from build123d import *

# Parameters (mm, degrees)
SKETCH1_W           = 65
SKETCH1_H           = 51.65
BOSS_EXTRUDE1_DEPTH = 1
CHAMFER1_SIZE       = 5
CUT_EXTRUDE2_REACH  = 43.523
SKETCH2_R           = 1.75
SKETCH3_W           = 25.5
SKETCH3_H           = 1
BOSS_EXTRUDE3_DEPTH = 1
CUT_EXTRUDE3_REACH  = 44.152
SKETCH4_R           = 0.5
LPATTERN1_COUNT     = 6
LPATTERN1_PITCH     = 2.54
LPATTERN1_COL_COUNT = 5
LPATTERN1_COL_PITCH = 2.54
SKETCH5_W           = 9
SKETCH5_H           = 3.35
BOSS_EXTRUDE4_DEPTH = 1
CUT_EXTRUDE4_DEPTH  = 0.2


with BuildPart() as part:
    # Sketch1 → Boss-Extrude1 (new body)
    with BuildSketch(Plane(origin=(0, 0, 0), x_dir=(1, 0, 0), z_dir=(0, 1, 0))):
        Rectangle(SKETCH1_W, SKETCH1_H)
    extrude(amount=BOSS_EXTRUDE1_DEPTH)

    # Chamfer1
    chamfer1_edges = [part.edges().sort_by_distance(p)[0] for p in [
        (-32.5, 0.5, -25.825),
        (32.5, 0.5, -25.825),
        (32.5, 0.5, 25.825),
        (-32.5, 0.5, 25.825),
    ]]
    chamfer(chamfer1_edges, length=CHAMFER1_SIZE)

    # Sketch2 → Cut-Extrude2 (cut, up to next)
    with BuildSketch(Plane(origin=(0, 0, 0), x_dir=(1, 0, 0), z_dir=(0, 1, 0)), mode=Mode.PRIVATE) as cut_extrude2_sk1:
        with Locations(Location((-25.3, 18.625, 0), (0, 0, 270))):
            Circle(SKETCH2_R)
    cut_extrude2_tool1 = extrude(cut_extrude2_sk1.sketch, amount=CUT_EXTRUDE2_REACH, mode=Mode.PRIVATE) & part.part
    # Sketch2 → Cut-Extrude2 (cut, up to next)
    with BuildSketch(Plane(origin=(0, 0, 0), x_dir=(1, 0, 0), z_dir=(0, 1, 0)), mode=Mode.PRIVATE) as cut_extrude2_sk2:
        with Locations(Location((25.3, 18.625, 0), (0, 0, 270))):
            Circle(SKETCH2_R)
    cut_extrude2_tool2 = extrude(cut_extrude2_sk2.sketch, amount=CUT_EXTRUDE2_REACH, mode=Mode.PRIVATE) & part.part
    add(cut_extrude2_tool1.solids().sort_by_distance((-25.3, 0, -18.625))[0], mode=Mode.SUBTRACT)
    add(cut_extrude2_tool2.solids().sort_by_distance((25.3, 0, -18.625))[0], mode=Mode.SUBTRACT)

    # Sketch3 → Boss-Extrude3 (add)
    with BuildSketch(Plane(origin=(0, 1, 0), x_dir=(1, 0, 0), z_dir=(0, 1, 0))):
        with Locations((0, 26.325)):
            Rectangle(SKETCH3_W, SKETCH3_H)
    extrude(amount=-BOSS_EXTRUDE3_DEPTH)

    # Sketch4 → Cut-Extrude3 (cut, up to next)
    with BuildSketch(Plane(origin=(0, 1, 0), x_dir=(1, 0, 0), z_dir=(0, 1, 0)), mode=Mode.PRIVATE) as cut_extrude3_sk1:
        with Locations(Location((-1.27, 25.825, 0), (0, 0, 270))):
            Circle(SKETCH4_R)
    cut_extrude3_tool1 = extrude(cut_extrude3_sk1.sketch, amount=-CUT_EXTRUDE3_REACH, mode=Mode.PRIVATE) & part.part
    cut_extrude3 = cut_extrude3_tool1.solids().sort_by_distance((-1.27, 1, -25.825))[0]
    add(cut_extrude3, mode=Mode.SUBTRACT)

    # LPattern1: Cut-Extrude3 ×6
    with Locations(*[(i * LPATTERN1_PITCH, 0, 0) for i in range(1, LPATTERN1_COUNT)]):
        add(cut_extrude3, mode=Mode.SUBTRACT)

    # LPattern1 col: Cut-Extrude3 ×5
    with Locations(*[(-i * LPATTERN1_COL_PITCH, 0, 0) for i in range(1, LPATTERN1_COL_COUNT)]):
        add(cut_extrude3, mode=Mode.SUBTRACT)

    # Sketch5 → Boss-Extrude4 (add)
    with BuildSketch(Plane(origin=(0, 1, 0), x_dir=(1, 0, 0), z_dir=(0, 1, 0))):
        with Locations((21.76, 27.5)):
            Rectangle(SKETCH5_W, SKETCH5_H)
    extrude(amount=-BOSS_EXTRUDE4_DEPTH)

    # Sketch6 → Cut-Extrude4 (cut)
    with BuildSketch(Plane(origin=(0, 1, 0), x_dir=(1, 0, 0), z_dir=(0, 1, 0))):
        with BuildLine():
            Line((25.8, 28.115), (25.8, 27.515))
            ThreePointArc((25.8, 27.515), (25.3, 27.015), (24.8, 27.515))
            Line((24.8, 27.515), (24.8, 28.115))
            ThreePointArc((24.8, 28.115), (25.3, 28.615), (25.8, 28.115))
        make_face()
    extrude(amount=-CUT_EXTRUDE4_DEPTH, mode=Mode.SUBTRACT)


solid = part.part
Geometry check sheet. Reference: the model listing, model coordinates, mm. Round coordinates to 2 decimals unless told otherwise and drop trailing zeros. Loops run counter-clockwise (first coordinate to the right, second up) from the corner with the lowest first, then second, coordinate; pieces in that order, holes last.
Item 1: Mould release check, pull along Z, two halves, no side actions. Record for faces 1 (the cylindrical face through (27.035, 0.493, -18.853)), 2 (the flat face through (-29.965, 0.493, -23.36)), 3 (the flat face through (30.035, 0.493, 23.29)): pulls with the +Z half, pulls with the -Z half, needs draft (parallel to the pull), parting line crosses it, or undercut.
Item 2: Thickness scan on line 1 (Z direction, x = -11.5, y = 0.45) (3 decimals); line 2 (Z direction, x = -23, y = 0.5) (3 decimals); line 3 (Z direction, x = 3, y = 0.6) (3 decimals). Record the ranges inside material, lowest first.
Item 3: Cross-section at B-B on y = 0.5. Count the separate pieces of the cut face and the enclosed holes in it, then the cut area to 3 significant figures.
Item 4: Cross-section at A-A on x = -25.3. Record the boundary of the cut face in (y, z) (3 decimals).
Item 5: Gauge pin test, flat end, axial feed: pin 1 (0.5 mm diameter, centred on x = 25.5, z = -27.5, fed in from +Y). Record the tip position at first contact, or that the pin passes through.
Item 6: Cross-section at C-C on x = -5. Record the boundary of the cut face in (y, z) (3 decimals), then the cut area to 4 significant figures.
Answer sheet:
1. face 1: undercut
1. face 2: pulls with the -Z half
1. face 3: pulls with the +Z half
2. line 1: z = -26.825 to -26.32, -25.33 to 25.825
2. line 2: z = -25.825 to 25.825
2. line 3: z = -26.825 to 25.825
3. separate pieces: 1
3. enclosed holes: 12
3. area: 3,340 mm2
4. outline: (0, -25.825) - (1, -25.825) - (1, -20.375) - (0, -20.375) - close; (0, -16.875) - (1, -16.875) - (1, 25.825) - (0, 25.825) - close
5. pin 1: stops at y = 0.8
6. outline: (0, -26.825) - (1, -26.825) - (1, 25.825) - (0, 25.825) - close
6. area: 52.65 mm2
